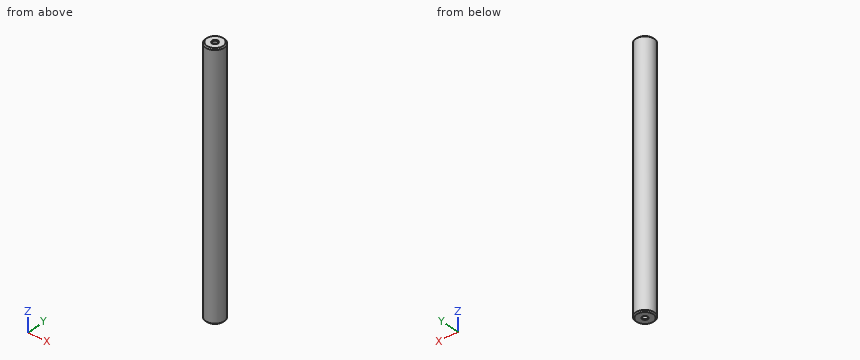
```python
from build123d import *

# Parameters (mm, degrees)
CHAMFER1_SIZE         = 0.5
CHAMFER2_SIZE         = 0.3
CHAMFER2_SIZE2        = 0.173205081
CHAMFER2_PART_2_SIZE  = 0.3
CHAMFER2_PART_2_SIZE2 = 0.173205081
CHAMFER2_PART_3_SIZE  = 0.3
CHAMFER2_PART_3_SIZE2 = 0.173205081
CHAMFER2_PART_4_SIZE  = 0.3
CHAMFER2_PART_4_SIZE2 = 0.173205081


with BuildPart() as part:
    # Sketch1 → Revolve1 (revolve)
    with BuildSketch(Plane(origin=(0, 0, 0), x_dir=(1, 0, 0), z_dir=(0, 1, 0))):
        Polygon((-1, 0), (-4, 0), (-4, -110), (-1, -110), (-1, -108), (0, -108), (0, -2), (-1, -2), align=None)
    revolve(axis=Axis((0, 0, 108), (0, 0, -1)))

    # Chamfer1
    chamfer1_edges = [part.edges().sort_by_distance(p)[0] for p in [
        (4, 0, 110),
        (4, 0, 0),
    ]]
    chamfer(chamfer1_edges, length=CHAMFER1_SIZE)

    # Chamfer2
    chamfer2_edges = [part.edges().sort_by_distance(p)[0] for p in [
        (1, 0, 2),
    ]]
    chamfer2_side = [part.faces().sort_by_distance(p)[0] for p in [
        (0, 0, 2),
    ]]
    chamfer(chamfer2_edges, length=CHAMFER2_SIZE, length2=CHAMFER2_SIZE2, reference=chamfer2_side[0])

    # Chamfer2 part 2
    chamfer2_part_2_edges = [part.edges().sort_by_distance(p)[0] for p in [
        (1, 0, 108),
    ]]
    chamfer2_part_2_side = [part.faces().sort_by_distance(p)[0] for p in [
        (1, 0, 109),
    ]]
    chamfer(chamfer2_part_2_edges, length=CHAMFER2_PART_2_SIZE, length2=CHAMFER2_PART_2_SIZE2, reference=chamfer2_part_2_side[0])

    # Chamfer2 part 3
    chamfer2_part_3_edges = [part.edges().sort_by_distance(p)[0] for p in [
        (1, 0, 110),
    ]]
    chamfer2_part_3_side = [part.faces().sort_by_distance(p)[0] for p in [
        (3.401005051, 0, 110),
    ]]
    chamfer(chamfer2_part_3_edges, length=CHAMFER2_PART_3_SIZE, length2=CHAMFER2_PART_3_SIZE2, reference=chamfer2_part_3_side[0])

    # Chamfer2 part 4
    chamfer2_part_4_edges = [part.edges().sort_by_distance(p)[0] for p in [
        (1, 0, 0),
    ]]
    chamfer2_part_4_side = [part.faces().sort_by_distance(p)[0] for p in [
        (1, 0, 1),
    ]]
    chamfer(chamfer2_part_4_edges, length=CHAMFER2_PART_4_SIZE, length2=CHAMFER2_PART_4_SIZE2, reference=chamfer2_part_4_side[0])


solid = part.part
```
Input: part model. Units: mm. Frame: model coordinates. Give positions to 0.01 mm unless a question says otherwise; leave off trailing zeros. Order: outer loops, then holes, each group sorted by start corner. A loop starts at its lowest first (then second) coordinate and runs counter-clockwise, first axis right, second up. Notation, with made-up numbers: (3, 58.5) - (44, 58.5) arc R25 ccw to (44, 89.5) - close; hole circle Ø4 at (51, 75.5). An arc over 180 degrees is marked (long way). One line per item, written item: value.
1. Line query: probe 1 along Y at (x, z) = (0, 109.5); probe 2 along X at (y, z) = (0.75, 28); probe 3 along Y at (x, z) = (2.25, 55). Output: solid intervals per line, ascending.
Determined:
probe 1: -4 to -1, 1 to 4
probe 2: -3.93 to 3.93
probe 3: -3.31 to 3.31
2. Pin query (flat end, axial travel): pin 1 Ø1.1 at (x, y) = (0.5, 0) entering from -Z; pin 2 Ø1.6 at (x, y) = (0, 0) entering from -Z; pin 3 Ø4 at (y, z) = (-3, 20.5) entering from -X. Return the tip coordinate at first contact, or that it passes through.
Determined:
pin 1: z = 0.21
pin 2: z = 1.94
pin 3: x = -3.87
3. Cut plane A-A, the plane z = 81.5. Output: boundary loops of the cut face in (x, y), and give its area (3 significant figures).
Determined:
outline: circle Ø8 at (0, 0)
area: 50.3 mm2
